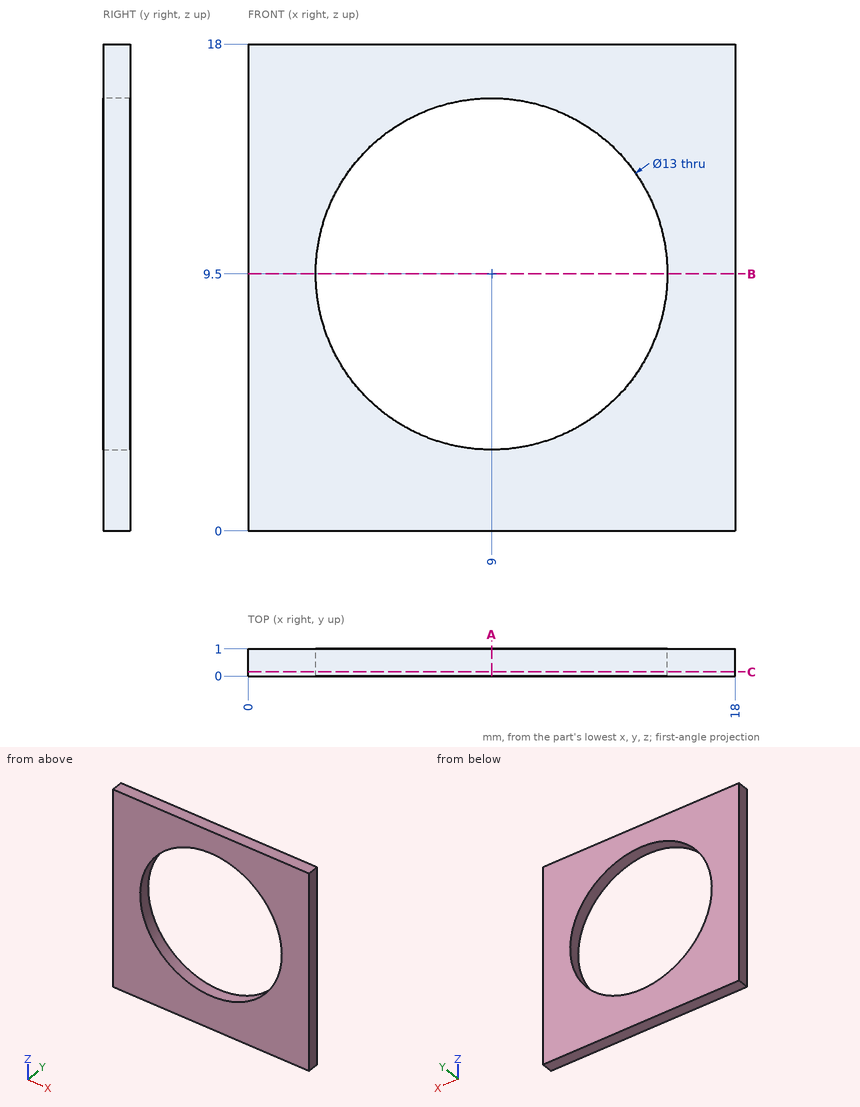
Drawing for the job (mm, zero at the part's lowest x, y, z). Round coordinates to 2 decimals unless told otherwise and drop trailing zeros. Write each loop counter-clockwise with the first axis right and the second up, starting at its lowest first coordinate (ties: lowest second). Pieces come first, ordered by that corner, then holes. Notation, with made-up numbers: M 37,-25 L 76,-25 A26 ccw 76,-4 Z; hole C 67.25,60.5 d8. An arc over 180 degrees is marked long. One line per question, with ' | ' between items.
1. Probe L1, parallel to X at y = 0.2, z = 9.75; L2, parallel to Z at x = 14.5, y = 0.6; L3, parallel to Z at x = 6, y = 0.2. List the from-to ranges inside material, lowest first. Write a range as from..to.
Working result:
L1: 0..2.5, 15.5..18 | L2: 0..6.04, 12.96..18 | L3: 0..3.73, 15.27..18
2. Pin check, flat tip, straight feed: pin 1 Ø1 at (x, z) = (4, 7.5) entering from +Y (1 decimal). Stop position of the tip, or through.
Working result:
pin 1: through
3. Cut at A-A on x = 9. Write the cut outline in (y, z), and give its area (3 significant figures).
Working result:
outline: M 0,0 L 1,0 L 1,3 L 0,3 Z; M 0,16 L 1,16 L 1,18 L 0,18 Z | area: 5.00 mm2
4. Cut at C-C on y = 0.15. Write the cut outline in (x, z), and give its area (3 significant figures).
Working result:
outline: M 0,0 L 18,0 L 18,18 L 0,18 Z; hole C 9,9.5 d13 | area: 191 mm2
5. Cut at B-B on z = 9.5. Write the cut outline in (x, y), and give its area (3 significant figures).
Working result:
outline: M 0,0 L 2.5,0 L 2.5,1 L 0,1 Z; M 15.5,0 L 18,0 L 18,1 L 15.5,1 Z | area: 5.00 mm2
